from build123d import *

# Parameters (mm, degrees)
SKETCH1_W           = 76.2
SKETCH1_H           = 25.4
SKETCH1_W_2         = 70.104
SKETCH1_H_2         = 19.304
BOSS_EXTRUDE1_DEPTH = 536.341159
CUT_EXTRUDE1_START  = -30.455423
SKETCH3_W           = 25.4
SKETCH3_H           = 76.2
CUT_EXTRUDE1_DEPTH  = 106.757864
CUT_EXTRUDE2_START  = -33.61888
SKETCH4_W           = 25.4
SKETCH4_H           = 76.2
CUT_EXTRUDE2_DEPTH  = 97.113932


with BuildPart() as part:
    # Sketch1 → Boss-Extrude1 (new body)
    with BuildSketch(Plane(origin=(0, 0, 0), x_dir=(1, 0, 0), z_dir=(0, 1, 0))):
        Rectangle(SKETCH1_W, SKETCH1_H)
        Rectangle(SKETCH1_W_2, SKETCH1_H_2, mode=Mode.SUBTRACT)
    extrude(amount=BOSS_EXTRUDE1_DEPTH)

    # Sketch3 → Cut-Extrude1 (cut)
    with BuildSketch(Plane(origin=(0, 536.341159245, 0), x_dir=(0, 0, -1), z_dir=(0.799354935, -0.600859125, 0)).offset(CUT_EXTRUDE1_START)):
        Rectangle(SKETCH3_W, SKETCH3_H)
    extrude(amount=CUT_EXTRUDE1_DEPTH, mode=Mode.SUBTRACT)

    # Sketch4 → Cut-Extrude2 (cut)
    with BuildSketch(Plane(origin=(0, 0, 0), x_dir=(0, 0, -1), z_dir=(0.882385297, 0.470527564, 0)).offset(CUT_EXTRUDE2_START)):
        Rectangle(SKETCH4_W, SKETCH4_H)
    extrude(amount=CUT_EXTRUDE2_DEPTH, mode=Mode.SUBTRACT)


solid = part.part
Can you work these out from the model? Positions are in its coordinate system, mm. A direction names the side the tool comes from. Give positions to 0.01 mm unless a question says otherwise; leave off trailing zeros. Loops run counter-clockwise (first coordinate to the right, second up) from the corner with the lowest first, then second, coordinate; pieces in that order, holes last. Notation, with made-up numbers: (37.25, 74.25) - (58.25, 74.25) arc R24 cw to (58.25, 87.25) - close; hole circle Ø8 at (20, -39.75). An arc over 180 degrees is marked (long way). Return JSON: item names as keys, results as strings.
1. I want a section at C-C on y = 226. Please give me the cut outline in (x, z).
Output values:
{"outline": "(-38.1, -12.7) - (38.1, -12.7) - (38.1, 12.7) - (-38.1, 12.7) - close; hole (-35.05, -9.65) - (35.05, -9.65) - (35.05, 9.65) - (-35.05, 9.65) - close"}
2. I want a section at A-A on z = 0. Please give me the cut outline in (x, y), and give its area (3 significant figures).
Output values:
{"outline": "(-38.1, 22.86) - (-35.05, 24.49) - (-35.05, 515.03) - (-38.1, 517.32) - close; (35.05, 61.87) - (38.1, 63.5) - (38.1, 460.04) - (35.05, 462.33) - close", "area": "2,720 mm²"}
3. For faces 5 (the face through (38.1, 259, 0)), 6 (the face through (-35.052, 266, 0)), which set-ups out of +Z, -Z, +X, -X, +Y, -Y let a thin tool reach every point of the face, with its end or its side?
Output values:
{"face 5": "+Z, -Z, +X, +Y, -Y", "face 6": "+Y, -Y"}
4. We'd pull the mould along X, two halves only. Please class faces 1 (the face through (-3, 41.58, 10.41)), 2 (the face through (-38.1, 267, 0)), 3 (the face through (35.052, 259, 0)), 4 (the face through (-1, 267, -12.7)): +X half, -X half, draft (parallel to the pull), parting line (faces both ways), or undercut.
Output values:
{"face 1": "+X half", "face 2": "-X half", "face 3": "undercut", "face 4": "draft"}
5. I want a section at B-B on x = -26.5. Please give me the cut outline in (y, z), and give its area (3 significant figures).
Output values:
{"outline": "(29.05, -12.7) - (508.6, -12.7) - (508.6, -9.65) - (29.05, -9.65) - close; (29.05, 9.65) - (508.6, 9.65) - (508.6, 12.7) - (29.05, 12.7) - close", "area": "2,920 mm²"}
6. If I drill on line 1 (Z direction, x = 18, y = 117); line 2 (X direction, y = 435, z = -2.5); line 3 (Y direction, x = 22, z = 11.5), over which ranges is the centre line in solid material (lowest first)?
Output values:
{"line 1": "z = -12.7 to -9.65, 9.65 to 12.7", "line 2": "x = -38.1 to -35.05, 35.05 to 38.1", "line 3": "y = 54.91 to 472.14"}
7. I'm going to push flat-ended pins straight in: pin 1 Ø10 at (x, z) = (-8, 5) entering from -Y; pin 2 Ø6 at (x, z) = (21, -7) entering from -Y. Where does each tip first touch, or does it pass through?
Output values:
{"pin 1": "stops at y = 37.94", "pin 2": "stops at y = 53.63"}
